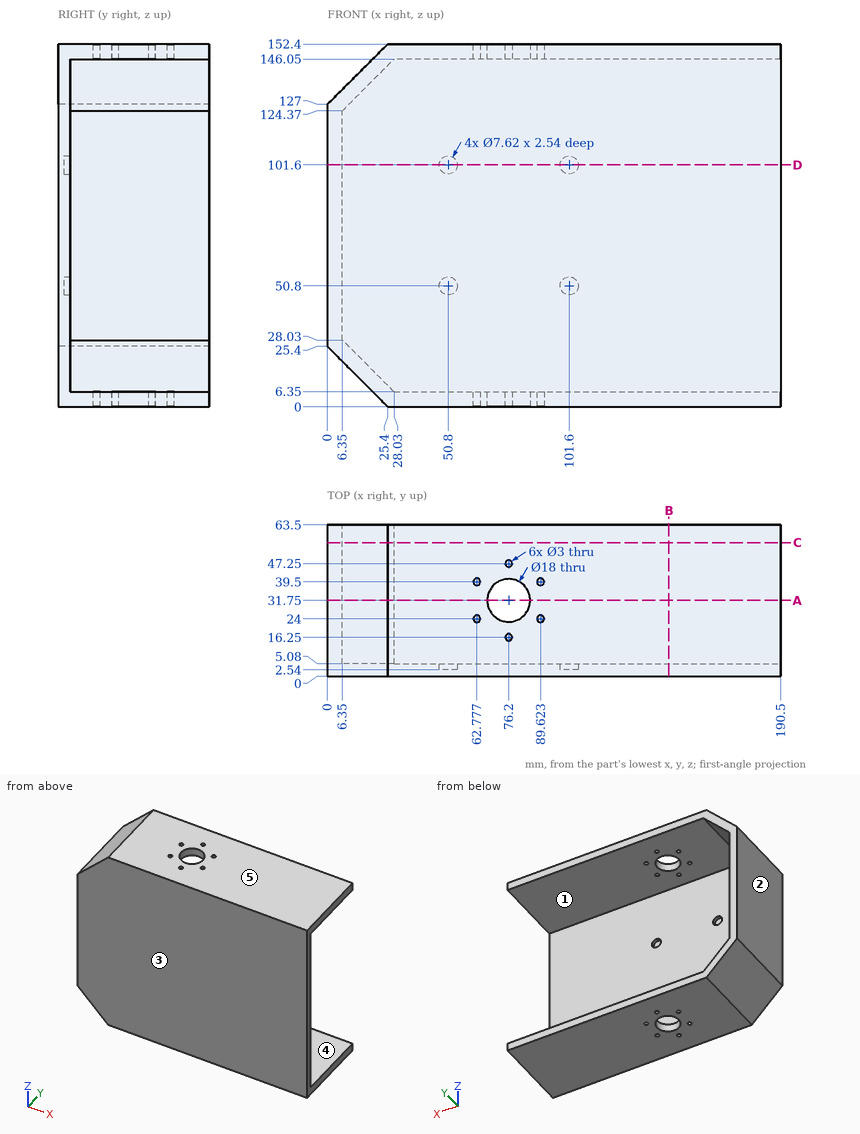
Answer from the drawing. Dimensions are ordinates in mm from the lowest x, y and z of the part. A direction names the side the tool comes from. Give positions to 0.01 mm unless a question says otherwise; leave off trailing zeros. Write each loop counter-clockwise with the first axis right and the second up, starting at its lowest first coordinate (ties: lowest second). Pieces come first, ordered by that corner, then holes. Notation, with made-up numbers: (-8, 44) - (51, 44) arc R33 cw to (51, 74) - close; hole circle Ø9 at (12.25, 9.5). An arc over 180 degrees is marked (long way). Answer in a Markdown table with one row per item. Add a question column.
Item 1: Section D-D, the plane z = 101.6 is taken. Write down the section's boundary in (x, y), and give its area (3 significant figures).
Item 2: Find the intervals of material crossed by L1, parallel to Z at x = 101, y = 4; L2, parallel to Z at x = 105.5, y = 11; L3, parallel to Y at x = 76, z = 2, in increasing order.
Item 3: Determine the mould class of the marked faces 3, 4 and 5 for opening direction Z: pulls with the +Z half, pulls with the -Z half, needs draft (parallel to the pull), parting line crosses it, or undercut.
Item 4: Section C-C, the plane y = 56 is taken. Write down the section's boundary in (x, z).
Item 5: Section B-B, the plane x = 143.5 is taken. Write down the section's boundary in (y, z).
Item 6: A tool of negligible diameter and unlimited length cuts with its end or side. For the marked faces 1 and 2, from which of +Z, -Z, +X, -X, +Y, -Y can it reach the whole face along a straight path? Write none if from no direction.
Item 7: Section A-A, the plane y = 31.75 is taken. Write down the section's boundary in (x, z), and give its area (3 significant figures).
Item 8: Flat-ended cylindrical pins translate along their axes: P1, Ø6, axis at x = 101.6, z = 50.8, coming from the +Y side; P2, Ø2, axis at y = 45, z = 131, coming from the +X side; P3, Ø12, axis at y = 28.5, z = 82, coming from the +X side. Find the tip coordinate at first contact, or state that the pin passes through.
Recorded:
| question | item | result |
|---|---|---|
| 1 | outline | (0, 0) - (190.5, 0) - (190.5, 5.08) - (105.41, 5.08) - (105.41, 2.54) - (97.79, 2.54) - (97.79, 5.08) - (54.61, 5.08) - (54.61, 2.54) - (46.99, 2.54) - (46.99, 5.08) - (6.35, 5.08) - (6.35, 63.5) - (0, 63.5) - close |
| 1 | area | 1,300 mm2 |
| 2 | L1 | z = 0 to 47.04, 54.56 to 97.84, 105.36 to 152.4 |
| 2 | L2 | z = 0 to 6.35, 146.05 to 152.4 |
| 2 | L3 | y = 0 to 14.76, 17.74 to 22.75, 40.75 to 45.76, 48.74 to 63.5 |
| 3 | face 3 | needs draft |
| 3 | face 4 | undercut |
| 3 | face 5 | pulls with the +Z half |
| 4 | outline | (0, 25.4) - (25.4, 0) - (190.5, 0) - (190.5, 6.35) - (28.03, 6.35) - (6.35, 28.03) - (6.35, 124.37) - (28.03, 146.05) - (190.5, 146.05) - (190.5, 152.4) - (25.4, 152.4) - (0, 127) - close |
| 5 | outline | (0, 0) - (63.5, 0) - (63.5, 6.35) - (5.08, 6.35) - (5.08, 146.05) - (63.5, 146.05) - (63.5, 152.4) - (0, 152.4) - close |
| 6 | face 1 | +X, +Y |
| 6 | face 2 | +Z, -Z, -X, +Y, -Y |
| 7 | outline | (0, 25.4) - (25.4, 0) - (67.2, 0) - (67.2, 6.35) - (28.03, 6.35) - (6.35, 28.03) - (6.35, 124.37) - (28.03, 146.05) - (67.2, 146.05) - (67.2, 152.4) - (25.4, 152.4) - (0, 127) - close; (85.2, 0) - (190.5, 0) - (190.5, 6.35) - (85.2, 6.35) - close; (85.2, 146.05) - (190.5, 146.05) - (190.5, 152.4) - (85.2, 152.4) - close |
| 7 | area | 2,900 mm2 |
| 8 | P1 | stops at y = 2.54 |
| 8 | P2 | stops at x = 13.98 |
| 8 | P3 | stops at x = 6.35 |
